Verification items for the finished model (mm, model axes). A direction names the side the tool comes from. Round coordinates to 2 decimals unless told otherwise and drop trailing zeros. Write each loop counter-clockwise with the first axis right and the second up, starting at its lowest first coordinate (ties: lowest second). Pieces come first, ordered by that corner, then holes. Notation, with made-up numbers: M 2,-3.5 L 15,-3.5 A25 ccw 15,22.5 Z; hole C 68.25,-7 d10. An arc over 180 degrees is marked long. One line per item, written item: value. Start each with the question number.
Item 1: Section check A-A, the plane z = 60. Record the cut outline in (x, y), then the cut area to 3 significant figures.
Item 2: Tool access check on faces 1 (the face through (-46, -30, 25)), 2 (the face through (-45, 0, 48)). Record the directions out of +Z, -Z, +X, -X, +Y, -Y that give a thin tool (end or side, any length) a straight path to the whole face; none if there is none.
Item 3: Thickness scan on probe 1 along Y at (x, z) = (-15, 1); probe 2 along X at (y, z) = (25.5, 16); probe 3 along Z at (x, y) = (-1.5, 24). Record the ranges inside material, lowest first. Write a range as from..to.
Item 4: Gauge pin test, flat ends, axial feed: pin 1 (5 mm diameter, centred on x = -40, y = 12.5, fed in from +Z); pin 2 (5 mm diameter, centred on y = -12.5, z = 21.5, fed in from +X); pin 3 (11.5 mm diameter, centred on x = -15, y = 15, fed in from -Z); pin 4 (1.5 mm diameter, centred on x = -41, y = 3, fed in from +Z). Record the tip position at first contact, or that the pin passes through.
Item 5: Section check D-D, the plane y = -24.5. Record the cut outline in (x, z).
Item 6: Section check B-B, the plane y = 15. Record the cut outline in (x, z), then the cut area to 3 significant figures.
Item 7: Draft check along Y on faces 3 (the face through (-46, 30, 25)), 4 (the face through (-18, 0, 5)), 5 (the face through (-16.08, 10.12, 0.07)). Enter one of: +Y half, -Y half, draft (parallel to the pull), parting line (faces both ways), or undercut.
Item 8: Section check C-C, the plane x = -15. Record the cut outline in (y, z).
from build123d import *

# Parameters (mm, degrees)
F0_W     = 60
F0_H     = 10
F3_R     = 10
F4_R     = 10
F5_DEPTH = 10.001
F6_R     = 5
F7_DEPTH = 25
F8_R     = 5
F9_DEPTH = 25


with BuildPart() as f2:
    # F2: sweep along a path in F1
    with BuildLine(Plane.XZ) as f2_path:
        Line((0, 0), (-50, 0))
        Line((-50, 0), (-50, 80))
    # F0 (on Right) → F2 (sweep)
    with BuildSketch(Plane.YZ):
        Rectangle(F0_W, F0_H)
    sweep(path=f2_path.line, transition=Transition.RIGHT)

    # F3
    f3_edges = [f2.edges().sort_by_distance(p)[0] for p in [
        (-45, 0, 5),
        (-55, 0, -5),
    ]]
    fillet(f3_edges, radius=F3_R)

    # F4 (on face) → F5 (cut, through all)
    with BuildSketch(Plane.YZ.offset(-45)):
        with Locations((0, 60)):
            Circle(F4_R)
    extrude(amount=-F5_DEPTH, mode=Mode.SUBTRACT)

    # F6 (on face) → F7 (cut)
    with BuildSketch(Plane.XY.offset(5)):
        with Locations((-15, 15)):
            Circle(F6_R)
    extrude(amount=-F7_DEPTH, mode=Mode.SUBTRACT)

    # F8 (on face) → F9 (cut)
    with BuildSketch(Plane.XY.offset(5)):
        with Locations((-15, -15)):
            Circle(F8_R)
    extrude(amount=-F9_DEPTH, mode=Mode.SUBTRACT)


solid = f2.part
Response values:
1. outline: M -55,-30 L -45,-30 L -45,-10 L -55,-10 Z; M -55,10 L -45,10 L -45,30 L -55,30 Z
1. area: 400 mm2
2. face 1: +Z, -Z, +X, -X, -Y
2. face 2: +Z, +X, +Y, -Y
3. probe 1: y = -30..-20, -10..10, 20..30
3. probe 2: x = -55..-45
3. probe 3: z = -5..5
4. pin 1: stops at z = 8.39
4. pin 2: stops at x = -45
4. pin 3: stops at z = -5
4. pin 4: stops at z = 7.62
5. outline: M -55,5 A10 ccw -45,-5 L 0,-5 L 0,5 L -35,5 A10 cw -45,15 L -45,80 L -55,80 Z
6. outline: M -55,5 A10 ccw -45,-5 L -20,-5 L -20,5 L -35,5 A10 cw -45,15 L -45,80 L -55,80 Z; M -10,-5 L 0,-5 L 0,5 L -10,5 Z
6. area: 1,200 mm2
7. face 3: +Y half
7. face 4: draft
7. face 5: undercut
8. outline: M -30,-5 L -20,-5 L -20,5 L -30,5 Z; M -10,-5 L 10,-5 L 10,5 L -10,5 Z; M 20,-5 L 30,-5 L 30,5 L 20,5 Z
